Can you work these out from the model? Positions are in its coordinate system, mm. Round coordinates to 2 decimals unless told otherwise and drop trailing zeros. Write each loop counter-clockwise with the first axis right and the second up, starting at its lowest first coordinate (ties: lowest second). Pieces come first, ordered by that corner, then holes.
Q1. If we section it at A-A (z = -0.05): Please give me the cut outline in (x, y).
Q2. If we section it at B-B (y = 43): Please give me the cut outline in (x, z) (3 decimals).
Q3. Please list where these lines run through material, in increasing order: line 1 along Y through (x, z) = (119.5, 0.05); line 2 along Y through (x, z) = (124, 0); line 3 along X through (y, z) = (47, -0.05).
Q4. If we section it at C-C (x = 85): Please give me the cut outline in (y, z) (3 decimals).
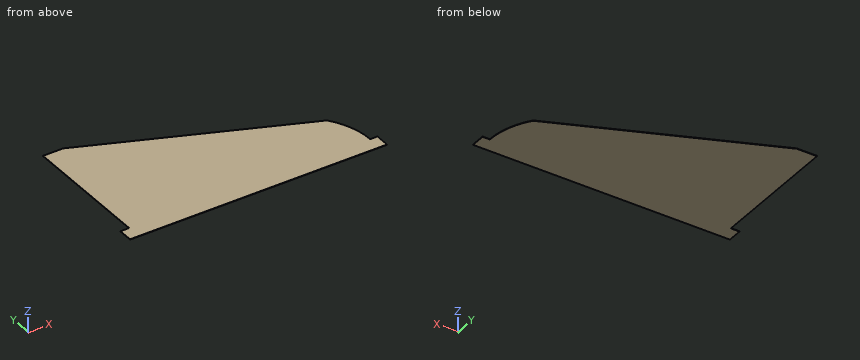
from build123d import *

# Parameters (mm, degrees)
BOSS_EXTRUDE1_DEPTH = 0.125
SKETCH2_W           = 1
SKETCH2_H           = 90
CUT_EXTRUDE1_DEPTH  = 200.822577553


with BuildPart() as part:
    # Sketch1 → Boss-Extrude1 (new, symmetric)
    with BuildSketch(Plane.XY):
        with BuildLine():
            Line((0, 0), (168, 0))
            Line((168, 0), (173, 0))
            Line((173, 0), (173, 10))
            Line((173, 10), (168, 10))
            ThreePointArc((168, 10), (165.434164903, 25.811388301), (158, 40))
            Line((158, 40), (15, 100))
            Line((15, 100), (0, 100))
            Line((0, 100), (0, 10))
            Line((0, 10), (-5, 10))
            Line((-5, 10), (-5, 0))
            Line((-5, 0), (0, 0))
        make_face()
    extrude(amount=BOSS_EXTRUDE1_DEPTH, both=True)

    # Sketch2 → Cut-Extrude1 (cut, through all)
    with BuildSketch(Plane.XY.offset(0.125)):
        with Locations((0.5, 55)):
            Rectangle(SKETCH2_W, SKETCH2_H)
    extrude(amount=-CUT_EXTRUDE1_DEPTH, mode=Mode.SUBTRACT)


solid = part.part
A:
1. outline: (-5, 0) - (173, 0) - (173, 10) - (168, 10) arc R50 ccw to (158, 40) - (15, 100) - (1, 100) - (1, 10) - (-5, 10) - close
2. outline: (1, -0.125) - (150.85, -0.125) - (150.85, 0.125) - (1, 0.125) - close
3. line 1: y = 0 to 56.15
3. line 2: y = 0 to 54.27
3. line 3: x = 1 to 141.32
4. outline: (0, -0.125) - (70.629, -0.125) - (70.629, 0.125) - (0, 0.125) - close
